For this review, use the dimensioned drawing (mm, ordinates from the lowest corner) and the shaded views. Round coordinates to 2 decimals unless told otherwise and drop trailing zeros. Loops run counter-clockwise (first coordinate to the right, second up) from the corner with the lowest first, then second, coordinate; pieces in that order, holes last. Notation, with made-up numbers: (89, 13) - (138, 13) arc R19 cw to (138, 38) - close; hole circle Ø7 at (-9, 84.5). An arc over 180 degrees is marked (long way). Use one line per item in the form item = value. Start each with the question number.
(1) For pin 1 (2 mm diameter, centred on x = 4.318, z = 6.731, fed in from +Y); pin 2 (0.6 mm diameter, centred on y = 3, z = 22.5, fed in from -X); pin 3 (1.5 mm diameter, centred on x = 0.5, z = 20.5, fed in from +Y); pin 4 (0.6 mm diameter, centred on y = 2.5, z = 21.5, fed in from +X) (1 decimal), all flat-tipped, find the tip position at first contact; note any pin that passes through.
(2) The part is to be moulded in two halves that separate along X. For the marked faces 1 and 2, say which applies: released by +X, released by -X, zero draft, split by the parting line, or undercut.
(3) We need section D-D, the plane z = 21. Write out the cut boundary in (x, y) (1 decimal).
(4) Wall thickness on probe 1 along Z at (x, y) = (4.25, 2.1); probe 2 along X at (y, z) = (2.15, 16.51) (1 decimal); probe 3 along Z at (x, y) = (3, 2.55) (1 decimal): over which ranges is each line inside the solid? List them lowest first. Write a range as [from, to].
(5) We need section A-A, the plane z = 16.51. Write out the cut boundary in (x, y) (1 decimal).
(6) We need section C-C, the plane y = 0.8. Write out the cut boundary in (x, z), then the cut area to 3 significant figures.
(7) We need section B-B, the plane x = 3.25. Write out the cut boundary in (y, z) (1 decimal).
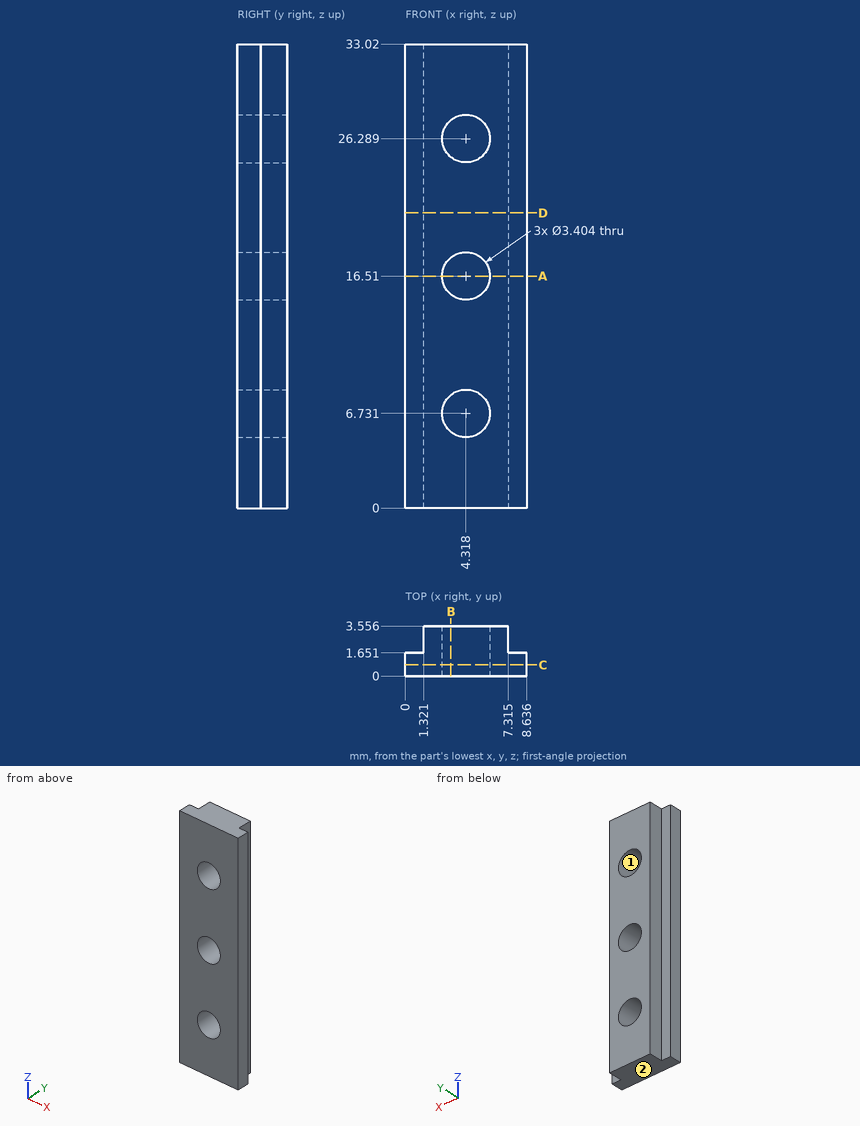
Data:
q1.pin_1 = through
q1.pin_2 = 1.32
q1.pin_3 = 1.65
q1.pin_4 = 7.3
q2.face_1 = undercut
q2.face_2 = zero draft
q3.outline = (0, 0) - (8.6, 0) - (8.6, 1.7) - (7.3, 1.7) - (7.3, 3.6) - (1.3, 3.6) - (1.3, 1.7) - (0, 1.7) - close
q4.probe_1 = [0, 5.03], [8.43, 14.81], [18.21, 24.59], [27.99, 33.02]
q4.probe_2 = [1.3, 2.6], [6, 7.3]
q4.probe_3 = [0, 5.7], [7.8, 15.4], [17.6, 25.2], [27.4, 33]
q5.outline = (0, 0) - (2.6, 0) - (2.6, 3.6) - (1.3, 3.6) - (1.3, 1.7) - (0, 1.7) - close; (6, 0) - (8.6, 0) - (8.6, 1.7) - (7.3, 1.7) - (7.3, 3.6) - (6, 3.6) - close
q6.outline = (0, 0) - (8.64, 0) - (8.64, 33.02) - (0, 33.02) - close; hole circle Ø3.4 at (4.32, 6.73); hole circle Ø3.4 at (4.32, 16.51); hole circle Ø3.4 at (4.32, 26.29)
q6.area = 258 mm^2
q7.outline = (0, 0) - (3.6, 0) - (3.6, 5.4) - (0, 5.4) - close; (0, 8.1) - (3.6, 8.1) - (3.6, 15.2) - (0, 15.2) - close; (0, 17.8) - (3.6, 17.8) - (3.6, 25) - (0, 25) - close; (0, 27.6) - (3.6, 27.6) - (3.6, 33) - (0, 33) - close
